from build123d import *

# Parameters (mm, degrees)
SKETCH2_R           = 1.27
CUT_EXTRUDE1_DEPTH  = 15.69747247
SKETCH3_R           = 17.78
SKETCH3_R_2         = 3.175
SKETCH3_R_3         = 1.55
BOSS_EXTRUDE1_DEPTH = 3.175


with BuildPart() as part:
    # Sketch1 → Revolve1 (revolve)
    with BuildSketch(Plane.XY, mode=Mode.PRIVATE) as revolve1_sk:
        Polygon((4.572, 0), (4.572, 1.905), (9.906, 1.905), (9.906, 4.445), (1.397, 4.445), (1.397, 2.54), (3.175, 2.54), (3.175, 0), align=None)
    revolve(revolve1_sk.sketch.rotate(Axis((0, 0, 0), (0, 1, 0)), 90), axis=Axis((0, 0, 0), (0, 1, 0)))

    # Sketch2 → Cut-Extrude1 (cut, through all)
    with BuildSketch(Plane(origin=(0, 4.445, 0), x_dir=(1, 0, 0), z_dir=(0, 1, 0))):
        with Locations(Location((0, 7, 0), (0, 0, 270))):
            Circle(SKETCH2_R)
        with Locations(Location((7, 0, 0), (0, 0, 270))):
            Circle(SKETCH2_R)
        with Locations(Location((0, -7, 0), (0, 0, 270))):
            Circle(SKETCH2_R)
        with Locations(Location((-7, 0, 0), (0, 0, 270))):
            Circle(SKETCH2_R)
    extrude(amount=-CUT_EXTRUDE1_DEPTH, mode=Mode.SUBTRACT)


with BuildPart() as body_2:
    # Sketch3 → Boss-Extrude1 (new body)
    with BuildSketch(Plane(origin=(0, 4.445, 0), x_dir=(1, 0, 0), z_dir=(0, 1, 0))):
        with Locations(Location((0, 0, 0), (0, 0, 270))):
            Circle(SKETCH3_R)
        with Locations(Location((0, 0, 0), (0, 0, 270))):
            Circle(SKETCH3_R_2, mode=Mode.SUBTRACT)
        with Locations(Location((-8.485281374, 8.485281374, 0), (0, 0, 270))):
            Circle(SKETCH3_R_3, mode=Mode.SUBTRACT)
        with Locations(Location((0, 7, 0), (0, 0, 270))):
            Circle(SKETCH3_R_3, mode=Mode.SUBTRACT)
        with Locations(Location((7, 0, 0), (0, 0, 270))):
            Circle(SKETCH3_R_3, mode=Mode.SUBTRACT)
        with Locations(Location((0, -7, 0), (0, 0, 270))):
            Circle(SKETCH3_R_3, mode=Mode.SUBTRACT)
        with Locations(Location((-7, 0, 0), (0, 0, 270))):
            Circle(SKETCH3_R_3, mode=Mode.SUBTRACT)
        with Locations(Location((8.485281374, 8.485281374, 0), (0, 0, 270))):
            Circle(SKETCH3_R_3, mode=Mode.SUBTRACT)
        with Locations(Location((8.485281374, -8.485281374, 0), (0, 0, 270))):
            Circle(SKETCH3_R_3, mode=Mode.SUBTRACT)
        with Locations(Location((-8.485281374, -8.485281374, 0), (0, 0, 270))):
            Circle(SKETCH3_R_3, mode=Mode.SUBTRACT)
    extrude(amount=BOSS_EXTRUDE1_DEPTH)


solid = body_2.part
Work out the finished part from the listing and answer in its coordinate system (mm). Coordinates: 2 decimals unless noted, no trailing zeros. Order: outer loops, then holes, each group sorted by start corner. A loop starts at its lowest first (then second) coordinate and runs counter-clockwise, first axis right, second up. Notation, with made-up numbers: (-22.5, 18) - (13.5, 18) arc R23 cw to (13.5, 34) - close; hole circle Ø8 at (5, 55). An arc over 180 degrees is marked (long way). Put each result on its own line as item: value. Start each with the question number.
1) Find the intervals of material crossed by line 1 (X direction, y = 6.9, z = 0) (3 decimals); line 2 (Z direction, x = 8, y = 6.4); line 3 (X direction, y = 6.3, z = 1), in increasing order. Write a range as from..to.
2) For a pull along Z with two mould halves and no side action, classify faces 1 (the cylindrical face through (-17.36, 6.01, -3.85)), 2 (the cylindrical face through (-8.513, 6.01, -0.336)), 3 (the flat face through (-4, 4.445, 0)) as released by +Z, released by -Z, zero draft, split by the parting line, or undercut.
3) Find section B-B (x = 0). Give the vertices of the cut face in (y, z) (3 decimals), plus the area to 3 significant figures.
4) Find section C-C (y = 6.35). State how many separate pieces and enclosed holes the cut face has, plus the area to 3 significant figures.
5) Find section A-A (z = 0). Give the vertices of the cut face in (x, y) (3 decimals), plus the area to 3 significant figures.
6) Flat-ended cylindrical pins translate along their axes: pin 1 (1.5 mm diameter, centred on x = -9, y = 5, fed in from +Z); pin 2 (1.5 mm diameter, centred on x = 11, y = 6.5, fed in from -Z). Find the tip coordinate at first contact, or state that the pin passes through.
7) Find section D-D (z = -13). Give the vertices of the cut face in (x, y) (3 decimals).
Results list:
1. line 1: x = -17.78..-8.55, -5.45..-3.175, 3.175..5.45, 8.55..17.78
1. line 2: z = -15.88..-9.96, -7.01..-1.18, 1.18..7.01, 9.96..15.88
1. line 3: x = -17.75..-8.18, -5.82..-3.01, 3.01..5.82, 8.18..17.75
2. face 1: split by the parting line
2. face 2: undercut
2. face 3: zero draft
3. outline: (4.445, -17.78) - (7.62, -17.78) - (7.62, -8.55) - (4.445, -8.55) - close; (4.445, -5.45) - (7.62, -5.45) - (7.62, -3.175) - (4.445, -3.175) - close; (4.445, 3.175) - (7.62, 3.175) - (7.62, 5.45) - (4.445, 5.45) - close; (4.445, 8.55) - (7.62, 8.55) - (7.62, 17.78) - (4.445, 17.78) - close
3. area: 73.1 mm^2
4. separate pieces: 1
4. enclosed holes: 9
4. area: 901 mm^2
5. outline: (-17.78, 4.445) - (-8.55, 4.445) - (-8.55, 7.62) - (-17.78, 7.62) - close; (-5.45, 4.445) - (-3.175, 4.445) - (-3.175, 7.62) - (-5.45, 7.62) - close; (3.175, 4.445) - (5.45, 4.445) - (5.45, 7.62) - (3.175, 7.62) - close; (8.55, 4.445) - (17.78, 4.445) - (17.78, 7.62) - (8.55, 7.62) - close
5. area: 73.1 mm^2
6. pin 1: stops at z = 15.75
6. pin 2: stops at z = -14.53
7. outline: (-12.13, 4.445) - (12.13, 4.445) - (12.13, 7.62) - (-12.13, 7.62) - close
